The drawing under review shows one solid part. Ordinate dimensions are in mm from its lowest x, y, z. A direction names the side the tool comes from. Coordinates: 2 decimals unless noted, no trailing zeros. Write each loop counter-clockwise with the first axis right and the second up, starting at its lowest first coordinate (ties: lowest second). Pieces come first, ordered by that corner, then holes.
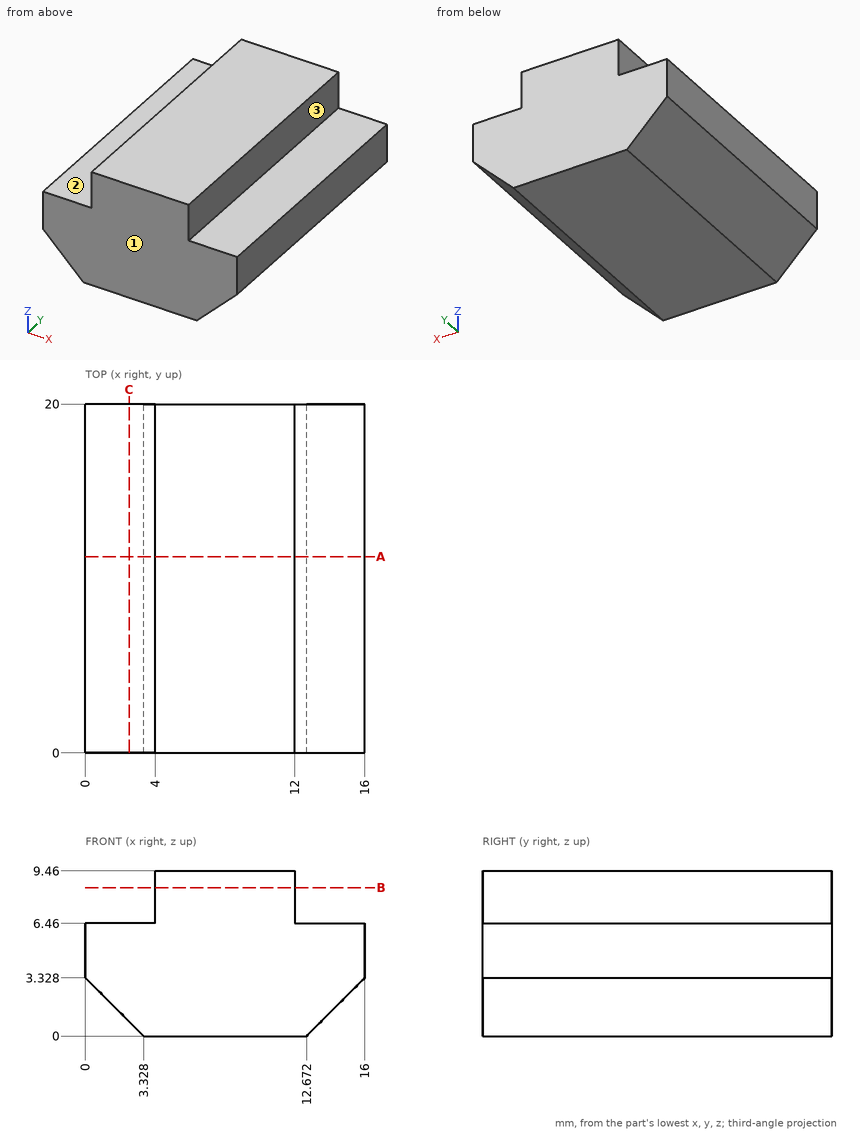
Q1. Add section A-A (y = 11.25). State the section outline as (x, z) points.
Ans:
outline: (0, 3.33) - (3.33, 0) - (12.67, 0) - (16, 3.33) - (16, 6.46) - (12, 6.46) - (12, 9.46) - (4, 9.46) - (4, 6.46) - (0, 6.46) - close
Q2. Add section C-C (x = 2.5). State the section outline as (y, z) points.
Ans:
outline: (0, 0.83) - (20, 0.83) - (20, 6.46) - (0, 6.46) - close
Q3. For probe 1 along X at (y, z) = (11.25, 9.25); probe 2 along Z at (x, y) = (15.25, 17.25); probe 3 along X at (y, z) = (8.5, 2.25), list the stretches that pass through material, from the lowest coordinate up.
Ans:
probe 1: x = 4 to 12
probe 2: z = 2.58 to 6.46
probe 3: x = 1.08 to 14.92
Q4. Add section B-B (z = 8.5). State the section outline as (x, y) points, then the cut area to 3 significant figures.
Ans:
outline: (4, 0) - (12, 0) - (12, 20) - (4, 20) - close
area: 160 mm2
Q5. Clearance check with flat-ended pins moving along their axes: pin 1 Ø3 at (x, y) = (1.5, 2.5) entering from -Z; pin 2 Ø2 at (x, y) = (2.5, 9) entering from +Z. State where each tip first meets the part, or that it passes through.
Ans:
pin 1: stops at z = 0.33
pin 2: stops at z = 6.46
Q6. Tool access review of the marked faces 1, 2 and 3: name each direction out of +Z, -Z, +X, -X, +Y, -Y from which nothing blocks a thin tool from reaching the whole face with its end or side.
Ans:
face 1: +Z, -Z, +X, -X, -Y
face 2: +Z, -X, +Y, -Y
face 3: +Z, +X, +Y, -Y
